The model under review builds one solid part; all positions refer to its coordinate system, in mm. A direction names the side the tool comes from. Give positions to 0.01 mm unless a question says otherwise; leave off trailing zeros. Loops run counter-clockwise (first coordinate to the right, second up) from the corner with the lowest first, then second, coordinate; pieces in that order, holes last. Notation, with made-up numbers: (-7.75, 43) -> (23.25, 43) arc R21 cw to (23.25, 48) -> close; hole circle Ø3 at (40, 67.5). An arc over 180 degrees is marked (long way). Write each question's results on one line, items separated by ' | '. Start each with the question number.
Q1. Machinability: for faces 1 (the face through (7, -10, 1)), 2 (the face through (47, -10, 1)), 3 (the face through (-10, 0, 1)), which of the approach directions +Z, -Z, +X, -X, +Y, -Y give a long, thin tool a straight path to every point of the face, cutting with its end or side? Answer none if there is none.
Q2. We need section C-C (y = -6). Write out the cut boundary in (x, z).
Q3. We need section B-B (x = 1). Write out the cut boundary in (y, z).
Q4. We need section D-D (z = 2.55). Write out the cut boundary in (x, y).
Q5. Wall thickness on L1, parallel to X at y = 0, z = 0.7; L2, parallel to Y at x = 60, z = 0.9; L3, parallel to X at y = 1, z = 2.55: over which ranges is each line inside the solid? List them lowest first. Write a range as [from, to].
Q6. Insertion check: pin 1 Ø6.5 at (x, y) = (60, 0) entering from -Z; pin 2 Ø8 at (x, y) = (37.58, -6) entering from -Z. Each pin has a flat end and moves straight along its axis. Give the tip position at first contact, or say it passes through.
Q7. Mouldability with a two-part tool opening along Y and no side actions: class faces 4 (the face through (3.905, -0.867, 1.521)), 5 (the face through (30, 10, 1)), 6 (the face through (29, -1, 0)) as released by +Y, released by -Y, zero draft, split by the parting line, or undercut.
Q8. We need section A-A (y = 0). Write out the cut boundary in (x, z).
Autodesk Inventor part; units mm, degrees
ref_plane "YZ Plane" through (0, 0, 0) normal (1, 0, 0) x (0, 1, 0)
ref_plane "XZ Plane" through (0, 0, 0) normal (0, 1, 0) x (-1, 0, 0)
ref_plane "XY Plane" through (0, 0, 0) normal (0, 0, 1) x (1, 0, 0)
sketch "Szkic1" plane through (0, 0, 0) normal (0, 0, 1) x (1, 0, 0)
  line L0 (0, 0) -> (60, 0) construction
  line L1 (0, -10) -> (14.7824, -10)
  line L2 (60, 10) -> (0, 10)
  arc A0 (0, 10) -> (0, -10) centre (0, 0) ccw
  arc A1 (60, -10) -> (60, 10) centre (60, 0) ccw
  arc A2 (30.2373, -10) -> (18.9235, -10) centre (24.5804, -12) ccw construction
  arc A3 (18.7016, -13.2) -> (30.4592, -13.2) centre (24.5804, -12) ccw
  line L3 (34.3784, -10) -> (60, -10)
  line L4 (18.9235, -10) -> (30.2373, -10)
  arc A4 (34.3784, -10) -> (30.4592, -13.2) centre (34.3784, -14) ccw
  arc A5 (18.7016, -13.2) -> (14.7824, -10) centre (14.7824, -14) ccw
  point P0 (30, 0)
  point P1 (37.5804, -6)
  point P2 (29.5804, -5)
  dimension "d0" = 60
  dimension "d1" = 20
  dimension "d20" = 12
  dimension "d21" = 4
  dimension "d22" = 13
  dimension "d23" = 6
  dimension "d24" = 30
  dimension "d25" = 1
  dimension "d26" = 8
  dimension "d27" = 5
extrude "Wyciągnięcie proste1" add sketch "Szkic1" along normal blind 3
hole "Otwór1" at (0, 0, 0) at (60, 0, 0) direction (0, 0, 1) diameter 8 end through all
hole "Otwór2" at (37.5804, -6, 0) at (24.5804, -12, 0) direction (0, 0, 1) diameter 5 end through all
properties part number "ramie_1_wahacza"
Output:
1) face 1: +Z, -Z, -X, -Y | face 2: +Z, -Z, +X, -Y | face 3: +Z, -Z, -X
2) outline: (-8, 0) -> (35.08, 0) -> (35.08, 3) -> (-8, 3) -> close; (40.08, 0) -> (68, 0) -> (68, 3) -> (40.08, 3) -> close
3) outline: (-10, 0) -> (-3.87, 0) -> (-3.87, 3) -> (-10, 3) -> close; (3.87, 0) -> (10, 0) -> (10, 3) -> (3.87, 3) -> close
4) outline: (0, -10) -> (14.78, -10) arc R4 cw to (18.7, -13.2) arc R6 ccw to (30.46, -13.2) arc R4 cw to (34.38, -10) -> (60, -10) arc R10 ccw to (60, 10) -> (0, 10) arc R10 ccw to start; hole circle Ø8 at (0, 0); hole circle Ø5 at (24.58, -12); hole circle Ø5 at (37.58, -6); hole circle Ø8 at (60, 0)
5) L1: [-10, -4], [4, 56], [64, 70] | L2: [-10, -4], [4, 10] | L3: [-9.95, -3.87], [3.87, 56.13], [63.87, 69.95]
6) pin 1: through | pin 2: z = 0
7) face 4: undercut | face 5: released by +Y | face 6: zero draft
8) outline: (-10, 0) -> (-4, 0) -> (-4, 3) -> (-10, 3) -> close; (4, 0) -> (56, 0) -> (56, 3) -> (4, 3) -> close; (64, 0) -> (70, 0) -> (70, 3) -> (64, 3) -> close
